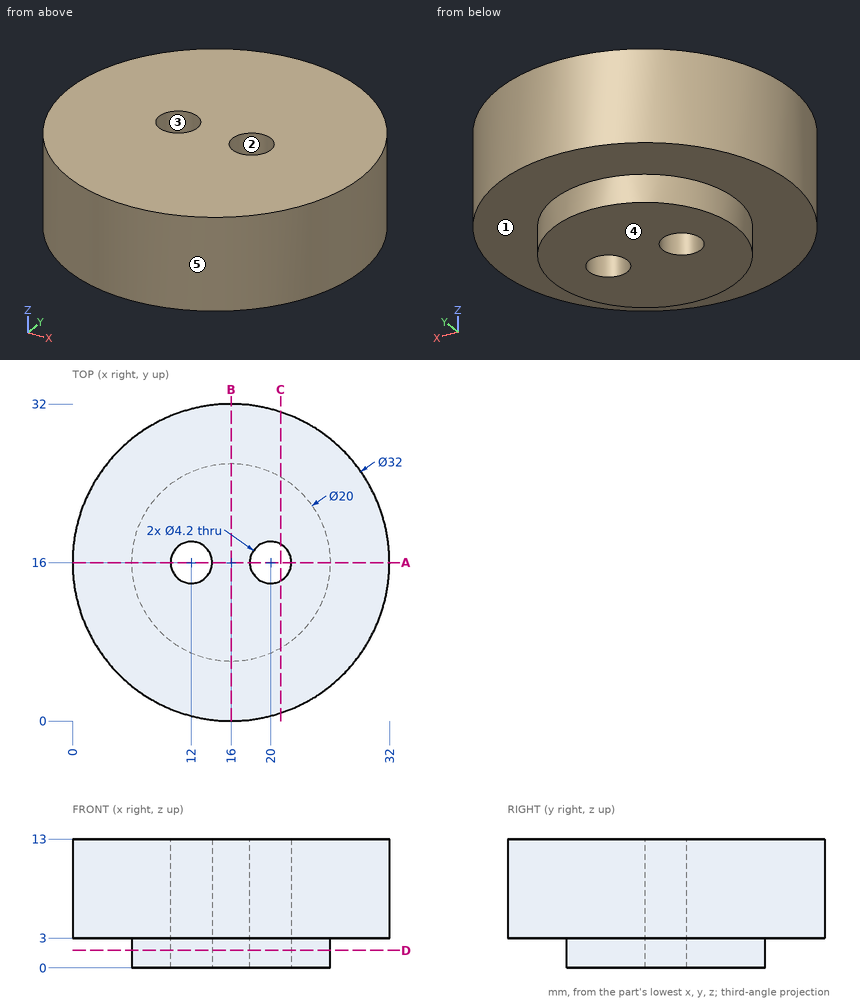
Job drawing, mm, ordinate dimensions from the low corner. One solid piece. A direction names the side the tool comes from. Coordinates: 2 decimals unless noted, no trailing zeros. Loops run counter-clockwise (first coordinate to the right, second up) from the corner with the lowest first, then second, coordinate; pieces in that order, holes last. Notation, with made-up numbers: (-32.75, -40) - (0.25, -40) arc R25 cw to (0.25, -12) - close; hole circle Ø6 at (61.5, 21.5). An arc over 180 degrees is marked (long way). Answer as a JSON object with one key per item and string values. Group by question number.
(1) Cut at C-C (x = 21). Give the cut face in (y, z), then the cut area to 3 significant figures.
(2) Probe line 1 along Z through (x, y) = (28, 23); line 2 along Y through (x, z) = (12, 5.5); line 3 along Y through (x, z) = (15.5, 7). List the from-to ranges inside material, lowest first.
(3) Two-plate mould, pull along Y, no slides. Class the marked faces 3, 4 and 5: released by +Y, released by -Y, zero draft, split by the parting line, or undercut.
(4) Cut at A-A (y = 16). Give the cut face in (x, z), then the cut area to 3 significant figures.
(5) Tool access for the marked faces 1 and 2: list every direction of +Z, -Z, +X, -X, +Y, -Y with a clear straight run to the whole face (end or side of a thin tool).
(6) Flat gauge pins, fed straight in: pin 1 (3.5 mm diameter, centred on x = 20, y = 16, fed in from -Z); pin 2 (2 mm diameter, centred on x = 12.5, z = 6.5, fed in from -Y); pin 3 (4 mm diameter, centred on y = 19.5, z = 8, fed in from -X); pin 4 (4 mm diameter, centred on x = 23, z = 4.5, fed in from +Y). Where does each tip first touch, or does it go through?
(7) Cut at B-B (x = 16). Give the cut face in (y, z), then the cut area to 3 significant figures.
(8) Cut at D-D (z = 1.75). Give the cut face in (x, y), then the cut area to 3 significant figures.
Geometry says:
{
 "1": {"outline": "(0.8, 3) - (7.34, 3) - (7.34, 0) - (14.15, 0) - (14.15, 13) - (0.8, 13) - close; (17.85, 0) - (24.66, 0) - (24.66, 3) - (31.2, 3) - (31.2, 13) - (17.85, 13) - close", "area": "308 mm^2"},
 "2": {"line 1": "z = 3 to 13", "line 2": "y = 0.51 to 13.9, 18.1 to 31.49", "line 3": "y = 0.01 to 31.99"},
 "3": {"face 3": "undercut", "face 4": "zero draft", "face 5": "split by the parting line"},
 "4": {"outline": "(0, 3) - (6, 3) - (6, 0) - (9.9, 0) - (9.9, 13) - (0, 13) - close; (14.1, 0) - (17.9, 0) - (17.9, 13) - (14.1, 13) - close; (22.1, 0) - (26, 0) - (26, 3) - (32, 3) - (32, 13) - (22.1, 13) - close", "area": "271 mm^2"},
 "5": {"face 1": "-Z", "face 2": "+Z, -Z"},
 "6": {"pin 1": "passes through", "pin 2": "stops at y = 0.2", "pin 3": "stops at x = 0.07", "pin 4": "stops at y = 31.2"},
 "7": {"outline": "(0, 3) - (6, 3) - (6, 0) - (26, 0) - (26, 3) - (32, 3) - (32, 13) - (0, 13) - close", "area": "380 mm^2"},
 "8": {"outline": "circle Ø20 at (16, 16); hole circle Ø4.2 at (12, 16); hole circle Ø4.2 at (20, 16)", "area": "286 mm^2"}
}
